Autodesk Inventor part; units mm, degrees
ref_plane "YZ Plane" through (0, 0, 0) normal (1, 0, 0) x (0, 1, 0)
ref_plane "XZ Plane" through (0, 0, 0) normal (0, 1, 0) x (-1, 0, 0)
ref_plane "XY Plane" through (0, 0, 0) normal (0, 0, 1) x (1, 0, 0)
sketch "Sketch1" plane through (0, 0, 0) normal (0, 0, 1) x (1, 0, 0)
  circle A0 centre (0, 0) radius 1.5
  dimension "d0" = 3
extrude "Extrusion1" add sketch "Sketch1" along normal blind 6
sketch "Sketch2" plane through (0, 0, 6) normal (0, 0, 1) x (1, 0, 0)
  circle A0 centre (0, 0) radius 2
  dimension "d3" = 4
extrude "Extrusion2" add sketch "Sketch2" along normal blind 36
sketch "Sketch3" plane through (0, 0, 42) normal (0, 0, 1) x (1, 0, 0)
  circle A0 centre (0, 0) radius 1.5
  dimension "d6" = 3
extrude "Extrusion3" add sketch "Sketch3" along normal blind 4
thread "Thread1"
properties material "Stainless Steel"
Source: CAD feature listing. Evaluate the final solid. Frame: model axes, mm. A direction names the side the tool comes from. Coordinates: 2 decimals unless noted, no trailing zeros. Loops run counter-clockwise (first coordinate to the right, second up) from the corner with the lowest first, then second, coordinate; pieces in that order, holes last. Notation, with made-up numbers: (17.25, -37.5) - (55.25, -37.5) arc R20 ccw to (55.25, -1.5) - close; hole circle Ø3 at (-24.75, 58.25). An arc over 180 degrees is marked (long way). One line per item, written item: value. Start each with the question number.
1. Section A-A (x = 0). Return the cut outline in (y, z).
2. Set-up query: faces 1 (the cylindrical face through (-1.5, -0.07, 43.97)), 2 (the cylindrical face through (-1.5, -0.07, 2.96)), 3 (the flat face through (0, 0, 46)). Return all of +Z, -Z, +X, -X, +Y, -Y with unobstructed straight access to the full face (end or side cutting, diameter ignored); none if empty.
3. Contact query for a flat-ended pin moving along its axis: P1, Ø1.5, axis at x = -1, z = 33.5, coming from the +Y side. Output: stop coordinate, or through.
4. Section C-C (z = 3.5). Return the cut outline in (x, y), and give its area (3 significant figures).
5. Ray query, L1, parallel to X at y = 0.15, z = 37; L2, parallel to Z at x = -0.55, y = 1.75; L3, parallel to X at y = -0.15, z = 2. Return the intervals inside material, ascending.
6. Section D-D (z = 19.5). Return the cut outline in (x, y), and give its area (3 significant figures).
Verdict:
1. outline: (-2, 6) - (-1.5, 6) - (-1.5, 0) - (1.5, 0) - (1.5, 6) - (2, 6) - (2, 42) - (1.5, 42) - (1.5, 46) - (-1.5, 46) - (-1.5, 42) - (-2, 42) - close
2. face 1: +Z
2. face 2: -Z
2. face 3: +Z, +X, -X, +Y, -Y
3. P1: stops at y = 1.98
4. outline: circle Ø3 at (0, 0)
4. area: 7.07 mm2
5. L1: x = -1.99 to 1.99
5. L2: z = 6 to 42
5. L3: x = -1.49 to 1.49
6. outline: circle Ø4 at (0, 0)
6. area: 12.6 mm2
